Geometry check sheet. Reference: drawing and pictorial views, mm from the part's lowest x, y, z. A direction names the side the tool comes from. Round coordinates to 2 decimals unless told otherwise and drop trailing zeros. Order: outer loops, then holes, each group sorted by start corner. A loop starts at its lowest first (then second) coordinate and runs counter-clockwise, first axis right, second up.
(1) Cross-section at D-D on y = 4.35. Enter the section's corners in (x, z) (3 decimals).
(2) Thickness scan on L1, parallel to X at y = 1, z = 6.5; L2, parallel to X at y = 4.5, z = 2.75; L3, parallel to Y at x = 9.75, z = 5.75. Record the ranges inside material, lowest first.
(3) Gauge pin test, flat ends, axial feed: P1, Ø3, axis at x = 13, z = 5.5, coming from the -Y side; P2, Ø1.6, axis at x = 10, z = 2.5, coming from the -Y side; P3, Ø3, axis at x = 5.035, y = 4.35, coming from the +Z side. Record the tip position at first contact, or that the pin passes through.
(4) Cross-section at B-B on y = 0.75. Enter the section's corners in (x, z), and give its area (3 significant figures).
(5) Draft check along X on the marked faces 1, 2, 3 and 4. Enter one of: pulls with the +X half, pulls with the -X half, needs draft (parallel to the pull), parting line crosses it, or undercut.
(6) Cross-section at A-A on z = 1.25. Enter the section's corners in (x, y) (3 decimals), and give its area (3 significant figures).
(7) Cross-section at C-C on x = 13.75. Enter the section's corners in (y, z), and give its area (3 significant figures).
(8) Set-up check for the marked faces 5 and 6: record each of +Z, -Z, +X, -X, +Y, -Y from which the full face is reachable in a straight line by a thin tool's end or side.
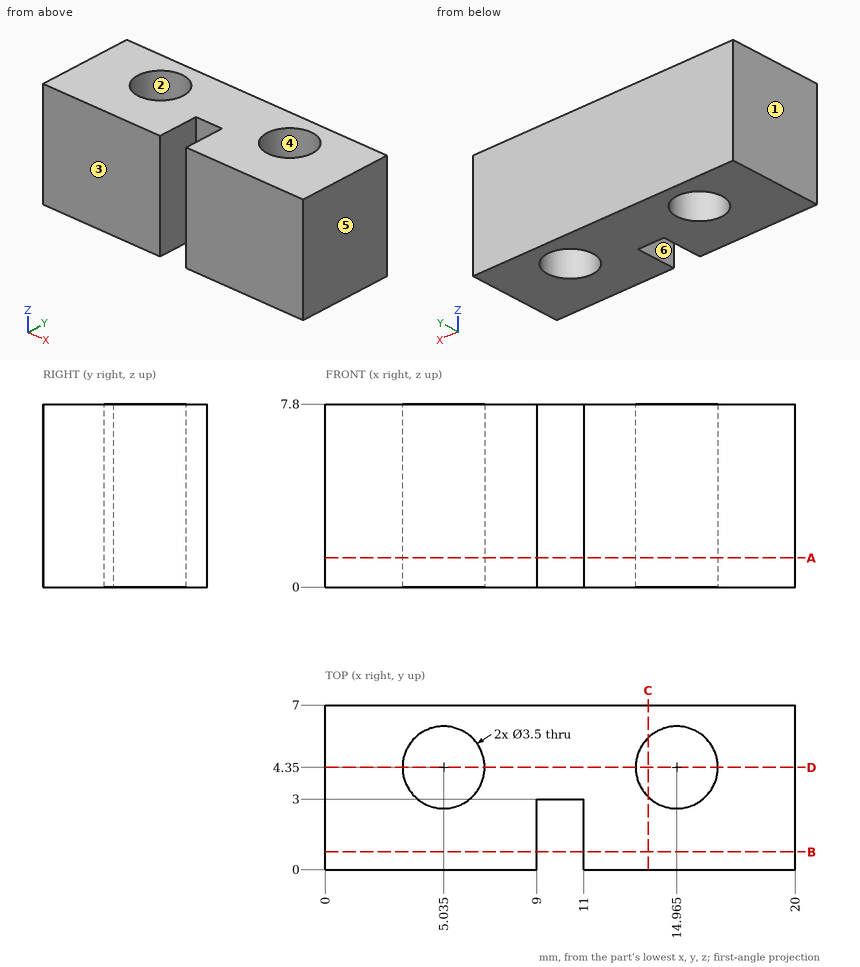
Found:
1. outline: (0, 0) - (3.285, 0) - (3.285, 7.8) - (0, 7.8) - close; (6.785, 0) - (13.215, 0) - (13.215, 7.8) - (6.785, 7.8) - close; (16.715, 0) - (20, 0) - (20, 7.8) - (16.715, 7.8) - close
2. L1: x = 0 to 9, 11 to 20
2. L2: x = 0 to 3.29, 6.78 to 13.22, 16.71 to 20
2. L3: y = 3 to 7
3. P1: stops at y = 0
3. P2: stops at y = 3
3. P3: passes through
4. outline: (0, 0) - (9, 0) - (9, 7.8) - (0, 7.8) - close; (11, 0) - (20, 0) - (20, 7.8) - (11, 7.8) - close
4. area: 140 mm2
5. face 1: pulls with the -X half
5. face 2: undercut
5. face 3: needs draft
5. face 4: undercut
6. outline: (0, 0) - (9, 0) - (9, 3) - (11, 3) - (11, 0) - (20, 0) - (20, 7) - (0, 7) - close; hole circle Ø3.5 at (5.035, 4.35); hole circle Ø3.5 at (14.965, 4.35)
6. area: 115 mm2
7. outline: (0, 0) - (3.09, 0) - (3.09, 7.8) - (0, 7.8) - close; (5.61, 0) - (7, 0) - (7, 7.8) - (5.61, 7.8) - close
7. area: 35.0 mm2
8. face 5: +Z, -Z, +X, +Y, -Y
8. face 6: +Z, -Z, -Y
